Work out the finished part from the listing and answer in its coordinate system (mm). Face numbers are marked on the shaded views. A direction names the side the tool comes from. Give positions to 0.01 mm unless a question says otherwise; leave off trailing zeros. Order: outer loops, then holes, each group sorted by start corner. A loop starts at its lowest first (then second) coordinate and runs counter-clockwise, first axis right, second up.
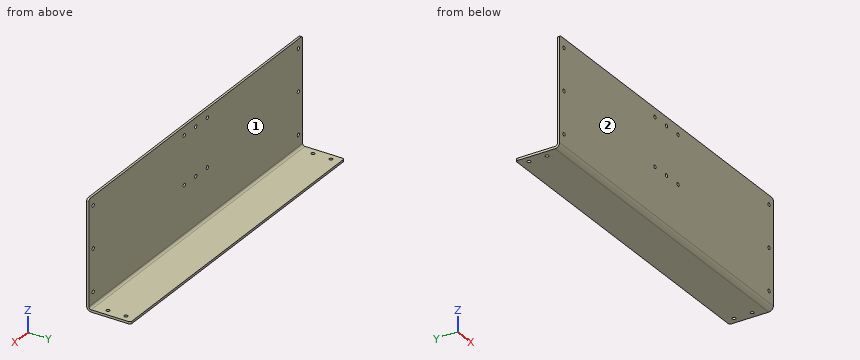
```python
from build123d import *

# Parameters (mm, degrees)
BASE_FLANGE1_DEPTH = 469.9
SKETCH6_R          = 21.9075
CUT_EXTRUDE1_DEPTH = 3.175
SKETCH7_R          = 2.4257
CUT_EXTRUDE2_DEPTH = 510.278313523
SKETCH8_R          = 2.4257
CUT_EXTRUDE3_DEPTH = 510.278313523
SKETCH9_R          = 2.4257
CUT_EXTRUDE4_DEPTH = 510.278313523
FILLET1_R          = 3.175
SKETCH10_W         = 152.4
SKETCH10_H         = 61.9125
CUT_EXTRUDE6_DEPTH = 510.278313523
FILLET2_R          = 3.175


# Sheet-metal steps are written as plain solids
with BuildPart() as part:
    # Sketch1 → Base-Flange1 (new body)
    with BuildSketch(Plane(origin=(0, 0, 0), x_dir=(0, 0, -1), z_dir=(1, 0, 0))):
        with BuildLine():
            Line((0, 0), (146.05, 0))
            ThreePointArc((146.05, 0), (150.540128061, 1.859871939), (152.4, 6.35))
            Line((152.4, 6.35), (152.4, 117.475))
            ThreePointArc((152.4, 117.475), (150.540128061, 121.965128061), (146.05, 123.825))
            Line((146.05, 123.825), (0, 123.825))
            Line((0, 123.825), (0, 120.65))
            Line((0, 120.65), (146.05, 120.65))
            ThreePointArc((146.05, 120.65), (148.29506403, 119.72006403), (149.225, 117.475))
            Line((149.225, 117.475), (149.225, 6.35))
            ThreePointArc((149.225, 6.35), (148.29506403, 4.10493597), (146.05, 3.175))
            Line((146.05, 3.175), (0, 3.175))
            Line((0, 3.175), (0, 0))
        make_face()
    extrude(amount=BASE_FLANGE1_DEPTH)

    # Sketch6 → Cut-Extrude1 (cut)
    with BuildSketch(Plane(origin=(0, 123.825, 0), x_dir=(1, 0, 0), z_dir=(0, 1, 0))):
        with Locations(Location((234.95, 46.0375, 0), (0, 0, 270))):
            Circle(SKETCH6_R)
    extrude(amount=-CUT_EXTRUDE1_DEPTH, mode=Mode.SUBTRACT)

    # Sketch7 → Cut-Extrude2 (cut, through all)
    with BuildSketch(Plane(origin=(0, 123.825, 0), x_dir=(1, 0, 0), z_dir=(0, 1, 0))):
        with Locations(Location((234.95, 12.2555, 0), (0, 0, 270))):
            Circle(SKETCH7_R)
        with Locations(Location((234.95, 79.8195, 0), (0, 0, 270))):
            Circle(SKETCH7_R)
        with Locations(Location((209.55, 12.2555, 0), (0, 0, 270))):
            Circle(SKETCH7_R)
        with Locations(Location((260.35, 12.2555, 0), (0, 0, 270))):
            Circle(SKETCH7_R)
        with Locations(Location((260.35, 79.8195, 0), (0, 0, 270))):
            Circle(SKETCH7_R)
        with Locations(Location((209.55, 79.8195, 0), (0, 0, 270))):
            Circle(SKETCH7_R)
    extrude(amount=-CUT_EXTRUDE2_DEPTH, mode=Mode.SUBTRACT)

    # Sketch8 → Cut-Extrude3 (cut, through all)
    with BuildSketch(Plane(origin=(0, 123.825, 0), x_dir=(1, 0, 0), z_dir=(0, 1, 0))):
        with Locations(Location((460.375, 12.7, 0), (0, 0, 270))):
            Circle(SKETCH8_R)
        with Locations(Location((460.375, 71.4375, 0), (0, 0, 270))):
            Circle(SKETCH8_R)
        with Locations(Location((460.375, 130.175, 0), (0, 0, 270))):
            Circle(SKETCH8_R)
        with Locations(Location((9.525, 130.175, 0), (0, 0, 270))):
            Circle(SKETCH8_R)
        with Locations(Location((9.525, 71.4375, 0), (0, 0, 270))):
            Circle(SKETCH8_R)
        with Locations(Location((9.525, 12.7, 0), (0, 0, 270))):
            Circle(SKETCH8_R)
    extrude(amount=-CUT_EXTRUDE3_DEPTH, mode=Mode.SUBTRACT)

    # Sketch9 → Cut-Extrude4 (cut, through all)
    with BuildSketch(Plane(origin=(0, 0, -152.4), x_dir=(-1, 0, 0), z_dir=(0, 0, -1))):
        with Locations((-460.375, 74.6125)):
            Circle(SKETCH9_R)
        with Locations((-460.375, 49.2125)):
            Circle(SKETCH9_R)
        with Locations((-9.525, 49.2125)):
            Circle(SKETCH9_R)
        with Locations((-9.525, 74.6125)):
            Circle(SKETCH9_R)
        with Locations((-460.375, 100.0125)):
            Circle(SKETCH9_R)
        with Locations((-460.375, 23.8125)):
            Circle(SKETCH9_R)
        with Locations((-9.525, 23.8125)):
            Circle(SKETCH9_R)
        with Locations((-9.525, 100.0125)):
            Circle(SKETCH9_R)
    extrude(amount=-CUT_EXTRUDE4_DEPTH, mode=Mode.SUBTRACT)

    # Fillet1
    fillet1_edges = [part.edges().sort_by_distance(p)[0] for p in [
        (0, 1.5875, 0),
        (0, 122.2375, 0),
        (469.9, 1.5875, 0),
        (469.9, 122.2375, 0),
    ]]
    fillet(fillet1_edges, radius=FILLET1_R)

    # Sketch10 → Cut-Extrude6 (cut, through all)
    with BuildSketch(Plane(origin=(469.9, 0, 0), x_dir=(0, 0, -1), z_dir=(1, 0, 0))):
        with Locations((76.2, 92.86875)):
            Rectangle(SKETCH10_W, SKETCH10_H)
    extrude(amount=-CUT_EXTRUDE6_DEPTH, mode=Mode.SUBTRACT)

    # Fillet2
    fillet2_edges = [part.edges().sort_by_distance(p)[0] for p in [
        (469.9, 61.9125, -150.8125),
        (0, 61.9125, -150.8125),
    ]]
    fillet(fillet2_edges, radius=FILLET2_R)


solid = part.part
```
1. Which of the six approach directions +Z, -Z, +X, -X, +Y, -Y give full straight-line access (tool end or side, diameter ignored) to the marked faces 1 and 2?
Findings below:
face 1: +Z, +X, -X, +Y
face 2: +Z, -Z, +X, -X, -Y
2. Straight lines are drawn through the part: probe 1 along X at (y, z) = (2, -12); probe 2 along Z at (x, y) = (260.35, 2.15); probe 3 along Y at (x, z) = (61.5, -60) (3 decimals). For each, find the intervals that lie inside material, in ascending order.
Findings below:
probe 1: x = 0 to 7.2, 11.85 to 207.14, 211.96 to 232.54, 237.36 to 257.94, 262.76 to 458.05, 462.7 to 469.9
probe 2: z = -150.81 to -82.25, -77.39 to -14.68, -9.83 to 0
probe 3: y = 0 to 3.175
3. The part is cut by section B-B (y = 37). Write down the section's boundary in (x, z) (3 decimals).
Findings below:
outline: (0, -152.4) - (469.9, -152.4) - (469.9, -149.225) - (0, -149.225) - close
4. The part is cut by section C-C (z = -36). Write down the section's boundary in (x, y) (3 decimals).
Findings below:
outline: (0, 0) - (469.9, 0) - (469.9, 3.175) - (0, 3.175) - close
5. Given P1, Ø3, axis at x = 260.35, z = -12.26, coming from the -Y side; P2, Ø3, axis at x = 131, z = -44, coming from the +Y side (3 decimals), each flat-ended and moving along its own axis, determine where each tip first touches the part or whether it passes through.
Findings below:
P1: passes through
P2: stops at y = 3.175
